Autodesk Fusion 360 part; units mm, degrees
sketch "Sketch1" plane through (0, 0, 0) normal (0, 0, 1) x (1, 0, 0)
  line L0 (-100, 100) -> (0, 100)
  line L1 (0, 100) -> (0, 0)
  line L2 (0, 0) -> (-100, 0)
  line L3 (-100, 0) -> (-100, 100)
extrude "Extrude1" add sketch "Sketch1" along normal blind 3 makes body 1
sketch "Sketch2" plane through (0, 0, 3) normal (0, 0, 1) x (-1, 0, 0)
  line L0 (100, 0) -> (0, 0)
  line L1 (0, 0) -> (0, -100)
  line L2 (0, -100) -> (100, -100)
  line L3 (100, -100) -> (100, 0)
  circle A0 centre (50, -50) radius 2.75
  dimension "d3" = 5.5
extrude "Extrude2" add sketch "Sketch2" along normal blind 1 contours L0 L1 L2 L3 | A0 bodies 1
sketch "Sketch3" plane through (0, 0, 4) normal (0, 0, 1) x (-1, 0, 0)
  line L0 (100, -100) -> (100, 0)
  line L1 (100, 0) -> (0, 0)
  line L2 (0, 0) -> (0, -100)
  line L3 (0, -100) -> (100, -100)
  circle A0 centre (50, -50) radius 2.75
  dimension "d6" = 5.5
extrude "Extrude3" cut sketch "Sketch3" against normal blind 3.25 contours A0 bodies 1
chamfer "Chamfer1" distance 0.5 angle 45 1 edges at (-47.4361, 49.0056, 4) on bodies 1
sketch "Sketch4" plane through (0, 0, 0) normal (0, 0, 1) x (1, 0, 0)
  line L0 (0, 0) -> (-25, 0)
  line L1 (-25, 0) -> (-25, 25)
  line L2 (-25, 25) -> (0, 25)
  line L3 (0, 25) -> (0, 0)
extrude "Extrude4" add sketch "Sketch4" along normal blind 3 separate body makes body 2
extrude "Extrude5" add 1 faces at (-8.3333, 8.3333, 3) along direction (0, 0, 1) blind 1 on bodies 2 bodies 2
sketch "Sketch5" plane through (0, 0, 4) normal (0, 0, 1) x (-1, 0, 0)
  line L0 (0, -25) -> (25, -25)
  line L1 (25, -25) -> (25, 0)
  line L2 (25, 0) -> (0, 0)
  line L3 (0, 0) -> (0, -25)
  circle A0 centre (12.5, -12.5) radius 2.75
  dimension "d14" = 5.5
extrude "Extrude6" cut sketch "Sketch5" against normal blind 3.25 contours A0 bodies 2
chamfer "Chamfer2" distance 0.5 angle 45 1 edges at (-9.9361, 11.5056, 4) on bodies 2
chamfer "Chamfer3" distance 0.5 angle 45 4 edges at (-12.5, 0, 4) (-25, 12.5, 4) (0, 12.5, 4) (-12.5, 25, 4) on bodies 2
sketch "Sketch6" plane through (0, 0, 4) normal (0, 0, 1) x (-1, 0, 0)
  circle A0 centre (12.5, -12.5) radius 3.25
  line L0 (0.5, -24.5) -> (24.5, -24.5)
  line L1 (24.5, -24.5) -> (24.5, -0.5)
  line L2 (24.5, -0.5) -> (0.5, -0.5)
  line L3 (0.5, -0.5) -> (0.5, -24.5)
  circle A1 centre (5, -5) radius 2.75
  circle A2 centre (20, -5) radius 2.75
  circle A3 centre (5, -20) radius 2.75
  circle A4 centre (20, -20) radius 2.75
  dimension "d19" = 5.5
  dimension "d20" = 5.5
  dimension "d21" = 5.5
  dimension "d22" = 5.5
extrude "Extrude7" cut sketch "Sketch6" against normal blind 3.25 contours A1 | A2 | A3 | A4 bodies 2
chamfer "Chamfer4" distance 0.5 angle 45 4 edges at (-2.4361, 4.0056, 4) (-17.4361, 4.0056, 4) (-17.4361, 19.0056, 4) (-2.4361, 19.0056, 4) on bodies 2
sketch "Sketch7" plane through (0, 0, 0) normal (0, 0, 1) x (1, 0, 0)
  line L0 (-25, 25) -> (0, 25)
  line L1 (0, 25) -> (0, 0)
  line L2 (0, 0) -> (-25, 0)
  line L3 (-25, 0) -> (-25, 25)
extrude "Extrude8" add sketch "Sketch7" along normal blind 3 separate body makes body 3
chamfer "Chamfer5" distance 1 angle 45 4 edges at (0, 25, 1.5) (0, 0, 1.5) (-25, 0, 1.5) (-25, 25, 1.5) on bodies 3
chamfer "Chamfer6" distance 0.5 angle 45 8 edges at (-0.5, 0.5, 3) (-12.5, 0, 3) (-24.5, 0.5, 3) (-25, 12.5, 3) (0, 12.5, 3) (-0.5, 24.5, 3) (-12.5, 25, 3) (-24.5, 24.5, 3) on bodies 3
sketch "Sketch8" plane through (0, 0, 3) normal (0, 0, 1) x (-1, 0, 0)
  line L0 (1.2071, -24.5) -> (23.7929, -24.5)
  line L1 (23.7929, -24.5) -> (24.5, -23.7929)
  line L2 (24.5, -23.7929) -> (24.5, -1.2071)
  line L3 (24.5, -1.2071) -> (23.7929, -0.5)
  line L4 (23.7929, -0.5) -> (1.2071, -0.5)
  line L5 (1.2071, -0.5) -> (0.5, -1.2071)
  line L6 (0.5, -1.2071) -> (0.5, -23.7929)
  line L7 (0.5, -23.7929) -> (1.2071, -24.5)
  circle A0 centre (12.5, -12.5) radius 2.25
  circle A1 centre (17, -17) radius 2.25
  circle A2 centre (8, -17) radius 2.25
  circle A3 centre (17, -8) radius 2.25
  circle A4 centre (8, -8) radius 2.25
  dimension "d30" = 4.5
  dimension "d31" = 4.5
  dimension "d32" = 4.5
  dimension "d33" = 4.5
  dimension "d34" = 4.5
extrude "Extrude9" cut sketch "Sketch8" against normal blind 2.2 contours A0 | A1 | A2 | A3 | A4 bodies 3
hidden bodies 1 2
Verification items for the finished model (mm, model axes). A direction names the side the tool comes from. Give positions to 0.01 mm unless a question says otherwise; leave off trailing zeros. Loops run counter-clockwise (first coordinate to the right, second up) from the corner with the lowest first, then second, coordinate; pieces in that order, holes last.
1. Thickness scan on line 1 (X direction, y = 8, z = 2.5); line 2 (Y direction, x = -8, z = 2); line 3 (Y direction, x = -12.5, z = 2.2). Record the ranges inside material, lowest first.
2. Section check B-B, the plane y = 17. Enter the section's corners in (x, z).
3. Section check A-A, the plane x = -12.5. Enter the section's corners in (y, z).
4. Section check D-D, the plane y = 11.75. Enter the section's corners in (x, z).
5. Mould release check, pull along Y, two halves, no side actions. Record for faces 3 (the flat face through (-0.5, 24.5, 1.2)), 4 (the flat face through (-24.32, 0.67, 2.75)), 5 (the cylindrical face through (-18.038, 18.996, 1.915)): released by +Y, released by -Y, zero draft, split by the parting line, or undercut.
6. Go/stop test with a flat-tipped pin: pin 1 Ø2 at (x, y) = (-17.5, 17) entering from +Z. Record where the tip stops, or that it passes through.
7. Section check C-C, the plane x = -17. Enter the section's corners in (y, z).
8. Set-up check for faces 1 (the flat face through (-17, 8, 0.8)), 2 (the flat face through (-25, 12, 1)): record each of +Z, -Z, +X, -X, +Y, -Y from which the full face is reachable in a straight line by a thin tool's end or side.
Geometry says:
1. line 1: x = -25 to -19.25, -14.75 to -10.25, -5.75 to 0
1. line 2: y = 0 to 5.75, 10.25 to 14.75, 19.25 to 25
1. line 3: y = 0 to 10.25, 14.75 to 25
2. outline: (-25, 0) - (0, 0) - (0, 2.5) - (-0.5, 3) - (-5.75, 3) - (-5.75, 0.8) - (-10.25, 0.8) - (-10.25, 3) - (-14.75, 3) - (-14.75, 0.8) - (-19.25, 0.8) - (-19.25, 3) - (-24.5, 3) - (-25, 2.5) - close
3. outline: (0, 0) - (25, 0) - (25, 2.5) - (24.5, 3) - (14.75, 3) - (14.75, 0.8) - (10.25, 0.8) - (10.25, 3) - (0.5, 3) - (0, 2.5) - close
4. outline: (-25, 0) - (0, 0) - (0, 2.5) - (-0.5, 3) - (-10.38, 3) - (-10.38, 0.8) - (-14.62, 0.8) - (-14.62, 3) - (-24.5, 3) - (-25, 2.5) - close
5. face 3: released by +Y
5. face 4: released by -Y
5. face 5: undercut
6. pin 1: stops at z = 0.8
7. outline: (0, 0) - (25, 0) - (25, 2.5) - (24.5, 3) - (19.25, 3) - (19.25, 0.8) - (14.75, 0.8) - (14.75, 3) - (10.25, 3) - (10.25, 0.8) - (5.75, 0.8) - (5.75, 3) - (0.5, 3) - (0, 2.5) - close
8. face 1: +Z
8. face 2: +Z, -Z, -X, +Y, -Y
